The model under review builds one solid part; all positions refer to its coordinate system, in mm. Face numbers are marked on the shaded views. A direction names the side the tool comes from. Round coordinates to 2 decimals unless told otherwise and drop trailing zeros. Write each loop counter-clockwise with the first axis right and the second up, starting at its lowest first coordinate (ties: lowest second). Pieces come first, ordered by that corner, then holes. Notation, with made-up numbers: M -14,61.5 L 22,61.5 A24 cw 22,84.5 Z; hole C -31.5,87 d5. An arc over 180 degrees is marked long. One line per item, written item: value. Start each with the question number.
1) Take a section at B-B, the plane x = 180. Write out the cut boundary in (y, z), and give its area (3 significant figures).
2) Take a section at D-D, the plane z = 2. Write out the cut boundary in (x, y), and give its area (3 significant figures).
3) For P1, Ø3, axis at x = 117.5, z = 15, coming from the -Y side; P2, Ø5.5, axis at x = 7, z = 6.5, coming from the +Y side; P3, Ø9.5, axis at x = 10, z = 10, coming from the -Y side; P4, Ø2, axis at y = 19, z = 3, coming from the -X side, all flat-tipped, find the tip position at first contact; note any pin that passes through.
4) Take a section at C-C, the plane y = 7.75. Write out the cut boundary in (x, z), and give its area (3 significant figures).
5) Mouldability with a two-part tool opening along X and no side actions: class the marked faces 4, 5 and 6 as +X half, -X half, draft (parallel to the pull), parting line (faces both ways), or undercut.
6) Take a section at A-A, the plane z = 10. Write out the cut boundary in (x, y).
7) Tool access review of the marked faces 1, 2 and 3: name each direction out of +Z, -Z, +X, -X, +Y, -Y from which nothing blocks a thin tool from reaching the whole face with its end or side.
8) Wall thickness on probe 1 along X at (y, z) = (-1.4, 10); probe 2 along X at (y, z) = (18.5, 8.5); probe 3 along X at (y, z) = (-2.35, 10): over which ranges is each line inside the solid? List them lowest first.
from build123d import *

# Parameters (mm, degrees)
EXTRUDE_THIN1_DEPTH = 20
FILLET1_R           = 1
CUT_EXTRUDE1_REACH  = 194.678
SKETCH2_R           = 3


with BuildPart() as part:
    # Sketch1 → Extrude-Thin1 (new body)
    with BuildSketch(Plane.XY):
        Polygon((0, 0), (20, 0), (20, 25), (170, 25), (170, 0), (190, 0), (190, -3), (167, -3), (167, 22), (23, 22), (23, -3), (0, -3), align=None)
    extrude(amount=EXTRUDE_THIN1_DEPTH)

    # Fillet1
    fillet1_edges = [part.edges().sort_by_distance(p)[0] for p in [
        (167, -3, 10),
        (23, -3, 10),
        (0, -3, 10),
        (0, 0, 10),
        (20, 25, 10),
        (170, 25, 10),
        (190, 0, 10),
        (190, -3, 10),
    ]]
    fillet(fillet1_edges, radius=FILLET1_R)

    # Sketch2 → Cut-Extrude1 (cut, up to next)
    with BuildSketch(Plane(origin=(0, 0, 0), x_dir=(1, 0, 0), z_dir=(0, 1, 0)), mode=Mode.PRIVATE) as cut_extrude1_sk1:
        with Locations(Location((10, -10, 0), (0, 0, 270))):
            Circle(SKETCH2_R)
    cut_extrude1_tool1 = extrude(cut_extrude1_sk1.sketch, amount=-CUT_EXTRUDE1_REACH, mode=Mode.PRIVATE) & part.part
    # Sketch2 → Cut-Extrude1 (cut, up to next)
    with BuildSketch(Plane(origin=(0, 0, 0), x_dir=(1, 0, 0), z_dir=(0, 1, 0)), mode=Mode.PRIVATE) as cut_extrude1_sk2:
        with Locations(Location((180, -10, 0), (0, 0, 270))):
            Circle(SKETCH2_R)
    cut_extrude1_tool2 = extrude(cut_extrude1_sk2.sketch, amount=-CUT_EXTRUDE1_REACH, mode=Mode.PRIVATE) & part.part
    add(cut_extrude1_tool1.solids().sort_by_distance((10, 0, 10))[0], mode=Mode.SUBTRACT)
    add(cut_extrude1_tool2.solids().sort_by_distance((180, 0, 10))[0], mode=Mode.SUBTRACT)


solid = part.part
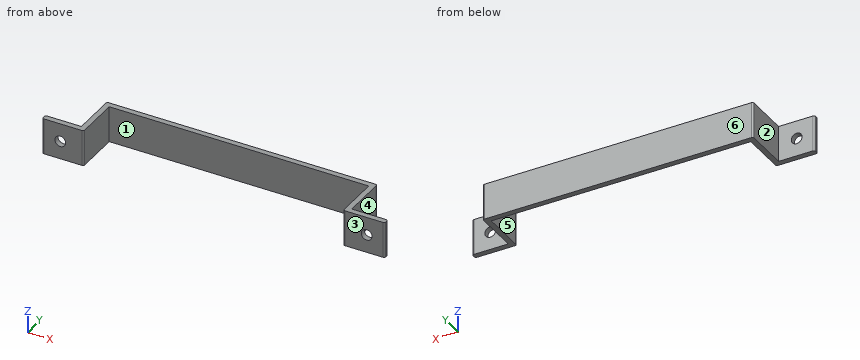
Checked values:
1. outline: M -3,0 L 0,0 L 0,7 L -3,7 Z; M -3,13 L 0,13 L 0,20 L -3,20 Z
1. area: 42.0 mm2
2. outline: M 0,-2 A1 ccw 1,-3 L 22,-3 A1 ccw 23,-2 L 23,22 L 167,22 L 167,-2 A1 ccw 168,-3 L 189,-3 A1 ccw 190,-2 L 190,-1 A1 ccw 189,0 L 170,0 L 170,24 A1 ccw 169,25 L 21,25 A1 ccw 20,24 L 20,0 L 1,0 A1 ccw 0,-1 Z
2. area: 718 mm2
3. P1: stops at y = 22
3. P2: stops at y = 0
3. P3: stops at y = -3
3. P4: stops at x = 20
4. outline: M 20,0 L 23,0 L 23,20 L 20,20 Z; M 167,0 L 170,0 L 170,20 L 167,20 Z
4. area: 120 mm2
5. face 4: +X half
5. face 5: undercut
5. face 6: draft
6. outline: M 0,-2 A1 ccw 1,-3 L 7,-3 L 7,0 L 1,0 A1 ccw 0,-1 Z; M 13,-3 L 22,-3 A1 ccw 23,-2 L 23,22 L 167,22 L 167,-2 A1 ccw 168,-3 L 177,-3 L 177,0 L 170,0 L 170,24 A1 ccw 169,25 L 21,25 A1 ccw 20,24 L 20,0 L 13,0 Z; M 183,-3 L 189,-3 A1 ccw 190,-2 L 190,-1 A1 ccw 189,0 L 183,0 Z
7. face 1: +Z, -Z, -Y
7. face 2: +Z, -Z, -X, +Y
7. face 3: +Z, -Z, +X, -X, -Y
8. probe 1: x = 0 to 7, 13 to 23, 167 to 177, 183 to 190
8. probe 2: x = 20 to 23, 167 to 170
8. probe 3: x = 0.06 to 7, 13 to 22.94, 167.06 to 177, 183 to 189.94
